Answer from the drawing. Dimensions are ordinates in mm from the lowest x, y and z of the part. Round coordinates to 2 decimals unless told otherwise and drop trailing zeros. Loops run counter-clockwise (first coordinate to the right, second up) from the corner with the lowest first, then second, coordinate; pieces in that order, holes last. Notation, with made-up numbers: M -28,83.25 L -5,83.25 A26 ccw -5,116.25 Z; hole C -27.5,28.5 d7. An arc over 180 degrees is marked long. Answer as CSV lines item,"result".
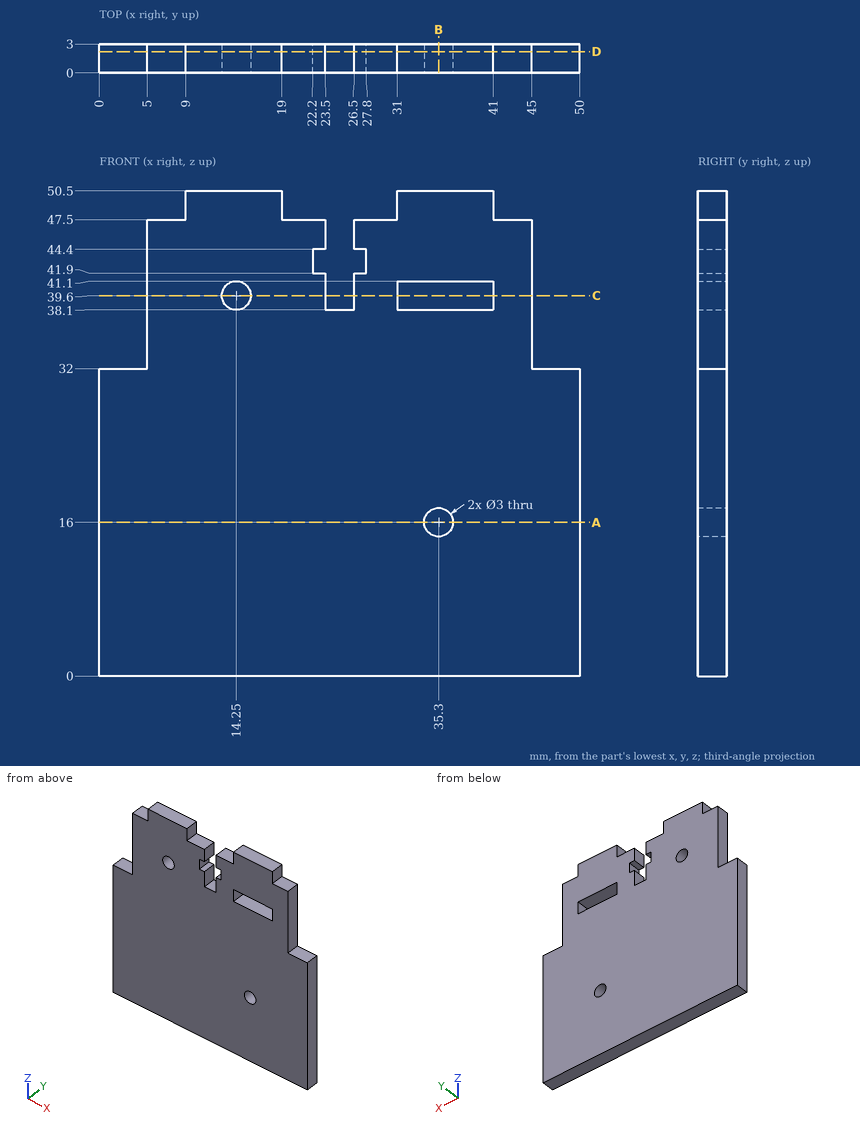
1) Find section A-A, the plane z = 16. Give the vertices of the cut face in (x, y), then the cut area to 3 significant figures.
Evaluation:
outline,"M 0,0 L 33.8,0 L 33.8,3 L 0,3 Z; M 36.8,0 L 50,0 L 50,3 L 36.8,3 Z"
area,"141 mm^2"
2) Each of these flat-tipped pins is pushed along its axis until it touches: P1, Ø5, axis at x = 28.5, z = 34, coming from the -Y side; P2, Ø0.9, axis at y = 1.5, z = 39.5, coming from the +X side; P3, Ø1.5, axis at x = 22, y = 1, coming from the +Z side; P4, Ø1.5, axis at y = 1.5, z = 46, coming from the -X side. Where does it stop, or does it pass through?
Evaluation:
P1,"stops at y = 0"
P2,"stops at x = 45"
P3,"stops at z = 47.5"
P4,"stops at x = 5"
3) Straight lines are drawn through the part: line 1 (X direction, y = 0.9, z = 39.6); line 2 (Z direction, x = 34, y = 2.65); line 3 (X direction, y = 1.5, z = 46). For each, find the intervals that lie inside material, in ascending order.
Evaluation:
line 1,"x = 5 to 12.75, 15.75 to 23.5, 26.5 to 31, 41 to 45"
line 2,"z = 0 to 15.25, 16.75 to 38.1, 41.1 to 50.5"
line 3,"x = 5 to 23.5, 26.5 to 45"
4) Find section C-C, the plane z = 39.6. Give the vertices of the cut face in (x, y), then the cut area to 3 significant figures.
Evaluation:
outline,"M 5,0 L 12.75,0 L 12.75,3 L 5,3 Z; M 15.75,0 L 23.5,0 L 23.5,3 L 15.75,3 Z; M 26.5,0 L 31,0 L 31,3 L 26.5,3 Z; M 41,0 L 45,0 L 45,3 L 41,3 Z"
area,"72.0 mm^2"
5) Find section D-D, the plane y = 2.2. Count the separate pieces of the cut face and the enclosed holes in it, then the cut area to 3 significant figures.
Evaluation:
separate pieces,"1"
enclosed holes,"3"
area,"2,200 mm^2"
6) Find section B-B, the plane x = 35.3. Give the vertices of the cut face in (y, z), then the cut area to 4 significant figures.
Evaluation:
outline,"M 0,0 L 3,0 L 3,14.5 L 0,14.5 Z; M 0,17.5 L 3,17.5 L 3,38.1 L 0,38.1 Z; M 0,41.1 L 3,41.1 L 3,50.5 L 0,50.5 Z"
area,"133.5 mm^2"
